Autodesk Inventor part; units mm, degrees
ref_plane "YZ Plane" through (0, 0, 0) normal (1, 0, 0) x (0, 1, 0)
ref_plane "XZ Plane" through (0, 0, 0) normal (0, 1, 0) x (-1, 0, 0)
ref_plane "XY Plane" through (0, 0, 0) normal (0, 0, 1) x (1, 0, 0)
sketch "Sketch1" plane through (0, 0, 0) normal (0, 0, 1) x (1, 0, 0)
  line L0 (126, -126) -> (-126, -126)
  line L1 (-126, -126) -> (-126, 126)
  line L2 (-126, 126) -> (126, 126)
  line L3 (126, 126) -> (126, -126)
  line L4 (126, -126) -> (-126, 126) construction
  line L5 (-126, -126) -> (126, 126) construction
  point P0 (0, 0)
  dimension "d0" = 252
  dimension "d1" = 252
extrude "Extrusion1" add sketch "Sketch1" along normal blind 6.35
sketch "Sketch2" plane through (0, 0, 6.35) normal (0, 0, 1) x (1, 0, 0)
  line L0 (-110.3923, 134) -> (-105.1962, 143)
  line L1 (-105.1962, 143) -> (-94.8038, 143)
  line L2 (-94.8038, 143) -> (-89.6077, 134)
  line L3 (-89.6077, 134) -> (-94.8038, 125)
  line L4 (-94.8038, 125) -> (-105.1962, 125)
  line L5 (-105.1962, 125) -> (-110.3923, 134)
  line L6 (94.8038, 143) -> (105.1962, 143)
  line L7 (105.1962, 143) -> (110.3923, 134)
  line L8 (110.3923, 134) -> (105.1962, 125)
  line L9 (105.1962, 125) -> (94.8038, 125)
  line L10 (94.8038, 125) -> (89.6077, 134)
  line L11 (89.6077, 134) -> (94.8038, 143)
  line L12 (-100, 134) -> (100, 134) construction
  line L13 (126, 126) -> (-126, 126)
  line L14 (-105.1962, 143) -> (-115.0111, 126)
  line L15 (105.1962, 143) -> (115.0111, 126)
  line L16 (94.8038, 143) -> (-94.8038, 143)
  line L17 (-126, -126) -> (126, -126)
  line L18 (-27.315, -126) -> (-17.5, -143)
  line L19 (-17.5, -143) -> (17.5, -143)
  line L20 (17.5, -143) -> (27.315, -126)
  line L21 (-70.1962, 143) -> (-60.3812, 126)
  line L22 (60.3812, 126) -> (70.1962, 143)
  point P0 (0, 0)
  point P1 (0, 134)
  point P2 (0, -143)
  point P3 (0, -134)
  dimension "d4" = 18
  dimension "d5" = 200
  dimension "d6" = 8
  dimension "d7" = 17
  dimension "d8" = 17
  dimension "d9" = 35
  dimension "d10" = 8
  dimension "d32" = 35
  dimension "d33" = 35
extrude "Extrusion2" add sketch "Sketch2" against normal up to surface (6.35 mm away) contours L0 L1 L2 L3 L13 L5 | L5 L13 L14 | L16 L21 L13 L3 L2 | L16 L11 L10 L13 L22 | L6 L7 L8 L13 L10 L11 | L8 L15 L13 | L17 L20 L19 L18
hole "Hole1" at (0, -134, 6.35) at (-100, 134, 6.35) at (100, 134, 6.35) direction (0, 0, -1) diameter 4.134 end through all
fillet "Fillet1" radius 2 16 edges at (17.5, -143, 3.175) (27.315, -126, 3.175) (126, -126, 3.175) (-126, 126, 3.175) (115.0111, 126, 3.175) (105.1962, 143, 3.175) (126, 126, 3.175) (-27.315, -126, 3.175) (-17.5, -143, 3.175) (-126, -126, 3.175) (-115.0111, 126, 3.175) (-105.1962, 143, 3.175) (-70.1962, 143, 3.175) (-60.3812, 126, 3.175) (60.3812, 126, 3.175) (70.1962, 143, 3.175)
sketch "Sketch3" plane through (0, 0, 6.35) normal (0, 0, 1) x (1, 0, 0)
  line L0 (150, -125) -> (-150, -125) construction
  line L1 (-150, -125) -> (-150, 125) construction
  line L2 (-150, 125) -> (150, 125) construction
  line L3 (150, 125) -> (150, -125) construction
  line L4 (150, -125) -> (-150, 125) construction
  line L5 (-150, -125) -> (150, 125) construction
  circle A0 centre (-75, 126.6) radius 1.6 construction
  line L6 (-75, 126.6) -> (75, 126.6) construction
  circle A1 centre (75, 126.6) radius 1.6 construction
  point P0 (0, 0)
  point P1 (0, 126.6)
  dimension "d21" = 300
  dimension "d22" = 250
  dimension "d23" = 3.2
  dimension "d24" = 150
hole "Hole2" at (-75, 126.6, 6.35) at (75, 126.6, 6.35) direction (0, 0, -1) diameter 2.459 end through all
equation "\"d7\" = d8"
equation "\"d32\" = d9"
equation "\"d33\" = d32"
properties part number "Print Bed" material "Aluminum 6061"
Check sheet for the modelled part. Datum: model origin and axes. Units: mm. A direction names the side the tool comes from. Round coordinates to 2 decimals unless told otherwise and drop trailing zeros. Loops run counter-clockwise (first coordinate to the right, second up) from the corner with the lowest first, then second, coordinate; pieces in that order, holes last. Notation, with made-up numbers: (-4, 80) -> (22, 80) arc R30 cw to (22, 105) -> close; hole circle Ø4 at (82.5, 20.5). An arc over 180 degrees is marked (long way). Answer in a Markdown table with one row per item.
Q1. Sectioned sample at A-A on z = 4.75. Give the number of separate pieces and of enclosed holes in the cut face, then the cut area to 3 significant figures.
Data:
| item | result |
|---|---|
| separate pieces | 1 |
| enclosed holes | 5 |
| area | 65,700 mm^2 |
Q2. Set-up check for faces 4 (the face through (-65.35, 134.61, 3.22)), 5 (the face through (77, -126, 3)), 6 (the face through (-120, 126, 3)), 7 (the face through (120, 126, 3)): record each of +Z, -Z, +X, -X, +Y, -Y from which the full face is reachable in a straight line by a thin tool's end or side.
Data:
| item | result |
|---|---|
| face 4 | +Z, -Z, +Y |
| face 5 | +Z, -Z, +X, -Y |
| face 6 | +Z, -Z, -X, +Y |
| face 7 | +Z, -Z, +X, +Y |
Q3. Thickness scan on L1, parallel to Y at x = 75, z = 2.5; L2, parallel to X at y = 126.6, z = 5; L3, parallel to Y at x = -100, z = 3. Record the ranges inside material, lowest first.
Data:
| item | result |
|---|---|
| L1 | y = -126 to 125.37, 127.83 to 143 |
| L2 | x = -114.74 to -76.23, -73.77 to -60.65, 60.65 to 73.77, 76.23 to 114.74 |
| L3 | y = -126 to 131.93, 136.07 to 143 |
Q4. Release check for a two-part mould opening along X. For faces 1 (the face through (65, 134, 3)), 2 (the face through (-76, -126, 3)), 3 (the face through (-22.47, -134.39, 3.22)) record: released by +X, released by -X, zero draft, split by the parting line, or undercut.
Data:
| item | result |
|---|---|
| face 1 | undercut |
| face 2 | zero draft |
| face 3 | released by -X |
Q5. Go/stop test with flat-tipped pins: P1, Ø2, axis at x = 86.5, z = 2, coming from the -Y side; P2, Ø3, axis at x = 75, y = 126.6, coming from the -Z side; P3, Ø1.9, axis at x = -120, z = 3, coming from the +Y side. Record where each tip stops, or that it passes through.
Data:
| item | result |
|---|---|
| P1 | stops at y = -126 |
| P2 | stops at z = 0 |
| P3 | stops at y = 126 |
Q6. Sectioned sample at B-B on x = -50.5. Enter the section's corners in (y, z).
Data:
| item | result |
|---|---|
| outline | (-126, 0) -> (126, 0) -> (126, 6.35) -> (-126, 6.35) -> close |
Q7. Sectioned sample at C-C on x = -23.5. Enter the section's corners in (y, z), then the cut area to 3 significant figures.
Data:
| item | result |
|---|---|
| outline | (-132.61, 0) -> (126, 0) -> (126, 6.35) -> (-132.61, 6.35) -> close |
| area | 1,640 mm^2 |
